```python
from build123d import *

# Parameters (mm, degrees)
SKETCH1_W           = 157
SKETCH1_H           = 18
BOSS_EXTRUDE1_DEPTH = 2
SKETCH2_W           = 20
SKETCH2_H           = 2
BOSS_EXTRUDE2_DEPTH = 17
SKETCH3_W           = 23
SKETCH3_H           = 18
BOSS_EXTRUDE3_DEPTH = 1


with BuildPart() as part:
    # Sketch1 → Boss-Extrude1 (new body)
    with BuildSketch(Plane.XY):
        with Locations((78.5, 9)):
            Rectangle(SKETCH1_W, SKETCH1_H)
    extrude(amount=BOSS_EXTRUDE1_DEPTH)

    # Sketch2 → Boss-Extrude2 (add)
    with BuildSketch(Plane(origin=(0, 0, 0), x_dir=(-1, 0, 0), z_dir=(0, 0, -1))):
        with Locations((-22, 9.9)):
            Rectangle(SKETCH2_W, SKETCH2_H)
    extrude(amount=BOSS_EXTRUDE2_DEPTH)

    # Sketch3 → Boss-Extrude3 (add)
    with BuildSketch(Plane(origin=(0, 0, -17), x_dir=(-1, 0, 0), z_dir=(0, 0, -1))):
        with Locations((-20.5, 9)):
            Rectangle(SKETCH3_W, SKETCH3_H)
    extrude(amount=BOSS_EXTRUDE3_DEPTH)


solid = part.part
```
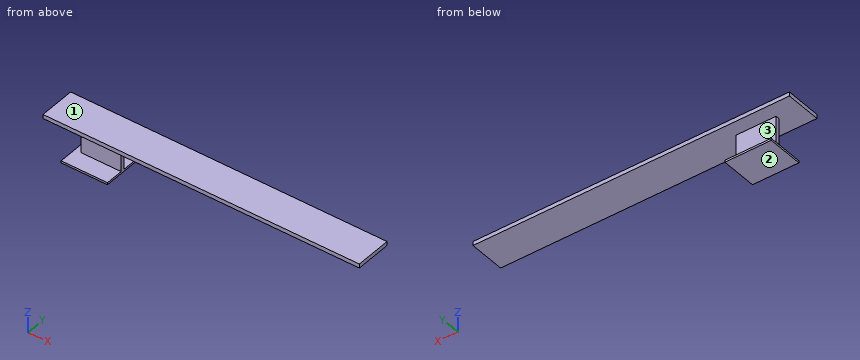
Build history of the part. All positions in model axes, mm. Face numbers are marked on the shaded views. Round coordinates to 2 decimals unless told otherwise and drop trailing zeros. Write each loop counter-clockwise with the first axis right and the second up, starting at its lowest first coordinate (ties: lowest second). Pieces come first, ordered by that corner, then holes.
1) Drill centre lines: probe 1 along Z at (x, y) = (12.5, 6); probe 2 along Z at (x, y) = (135, 14.25). Where is each one in solid material? Low to high.
2) Band-saw the part on D-D, the plane x = 116. List the corners of the cut face in (y, z), and give its area (3 significant figures).
3) Band-saw the part on B-B, the plane x = 18.5. List the corners of the cut face in (y, z).
4) Band-saw the part on C-C, the plane z = -3.5. List the corners of the cut face in (x, y), and give its area (3 significant figures).
5) Pin check, flat tips, straight feed: pin 1 (8 mm diameter, centred on x = 93, y = 15.5, fed in from -Z); pin 2 (1 mm diameter, centred on y = 6.5, z = -2.5, fed in from +X); pin 3 (5 mm diameter, centred on y = 9, z = -5, fed in from +X); pin 4 (1.5 mm diameter, centred on x = 26, z = -5, fed in from -Y). Stop position of each tip, or through.
6) Mould opens along Z. For the marked faces 1, 2 and 3 say: +Z half, -Z half, draft (parallel to the pull), parting line (faces both ways), or undercut.
7) Band-saw the part on A-A, the plane y = 6.25. List the corners of the cut face in (x, z), and give its area (3 significant figures).
Ans:
1. probe 1: z = -18 to -17, 0 to 2
1. probe 2: z = 0 to 2
2. outline: (0, 0) - (18, 0) - (18, 2) - (0, 2) - close
2. area: 36.0 mm2
3. outline: (0, -18) - (18, -18) - (18, -17) - (10.9, -17) - (10.9, 0) - (18, 0) - (18, 2) - (0, 2) - (0, 0) - (8.9, 0) - (8.9, -17) - (0, -17) - close
4. outline: (12, 8.9) - (32, 8.9) - (32, 10.9) - (12, 10.9) - close
4. area: 40.0 mm2
5. pin 1: stops at z = 0
5. pin 2: passes through
5. pin 3: stops at x = 32
5. pin 4: stops at y = 8.9
6. face 1: +Z half
6. face 2: -Z half
6. face 3: undercut
7. outline: (0, 0) - (157, 0) - (157, 2) - (0, 2) - close; (9, -18) - (32, -18) - (32, -17) - (9, -17) - close
7. area: 337 mm2
